Build history of the part. All positions in model axes, mm. Face numbers are marked on the shaded views. A direction names the side the tool comes from. Round coordinates to 2 decimals unless told otherwise and drop trailing zeros. Loops run counter-clockwise (first coordinate to the right, second up) from the corner with the lowest first, then second, coordinate; pieces in that order, holes last. Notation, with made-up numbers: (-36, 75.25) - (18, 75.25) arc R36 ccw to (18, 110.25) - close; hole circle Ø8 at (80, -10). An arc over 180 degrees is marked (long way). Use a Markdown table: item, result.
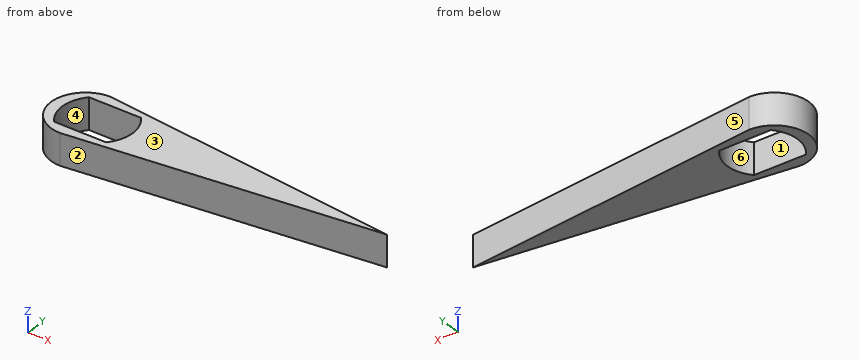
from build123d import *

# Parameters (mm, degrees)
PAD_DEPTH    = 2
POCKET_DEPTH = 2


with BuildPart() as part:
    # Sketch → Pad (new body)
    with BuildSketch(Plane(origin=(0, 0, 0), x_dir=(1, 0, 0), z_dir=(0, 0, -1))):
        with BuildLine():
            Line((0, 2.2), (19.5, 0))
            Line((19.5, 0), (0, -2.2))
            ThreePointArc((0, 2.2), (-2.2, 0), (0, -2.2))
        make_face()
    extrude(amount=PAD_DEPTH)

    # Sketch001 → Pocket (cut)
    with BuildSketch(Plane(origin=(0, 0, -2), x_dir=(1, 0, 0), z_dir=(0, 0, -1))):
        with BuildLine():
            Line((-0.899765, 1.5), (2.454335, 1.5))
            ThreePointArc((2.454335, -1.5), (3.027284, 0), (2.454335, 1.5))
            Line((-0.899765, -1.5), (2.454335, -1.5))
            ThreePointArc((-0.899765, 1.5), (-1.472714, 0), (-0.899765, -1.5))
        make_face()
    extrude(amount=-POCKET_DEPTH, mode=Mode.SUBTRACT)


solid = part.part
Q1. Pull direction Y, two halves, no side cores. Call the marked faces 3, 4, 5 and 6: pulls with the +Y half, pulls with the -Y half, needs draft (parallel to the pull), parting line crosses it, or undercut.
Results found:
| item | result |
|---|---|
| face 3 | needs draft |
| face 4 | undercut |
| face 5 | pulls with the +Y half |
| face 6 | undercut |
Q2. Cut at B-B, the plane y = 0.35. List the corners of the cut face in (x, z), plus the area to 3 significant figures.
Results found:
| item | result |
|---|---|
| outline | (-2.17, -2) - (-1.45, -2) - (-1.45, 0) - (-2.17, 0) - close; (3, -2) - (16.4, -2) - (16.4, 0) - (3, 0) - close |
| area | 28.2 mm2 |
Q3. Cut at D-D, the plane y = -0.6. List the corners of the cut face in (x, z), plus the area to 3 significant figures.
Results found:
| item | result |
|---|---|
| outline | (-2.12, -2) - (-1.39, -2) - (-1.39, 0) - (-2.12, 0) - close; (2.95, -2) - (14.18, -2) - (14.18, 0) - (2.95, 0) - close |
| area | 23.9 mm2 |
Q4. Probe line 1 (Y direction, x = 1, z = -1.3); line 2 (Y direction, x = 18.75, z = -1.75); line 3 (Y direction, x = 6.5, z = -0.05). List the from-to ranges inside material, lowest first.
Results found:
| item | result |
|---|---|
| line 1 | y = -2.09 to -1.5, 1.5 to 2.09 |
| line 2 | y = -0.08 to 0.08 |
| line 3 | y = -1.47 to 1.47 |
Q5. Cut at C-C, the plane y = 1.95. List the corners of the cut face in (x, z).
Results found:
| item | result |
|---|---|
| outline | (-1.02, -2) - (2.22, -2) - (2.22, 0) - (-1.02, 0) - close |
Q6. Cut at A-A, the plane z = -0.55. List the corners of the cut face in (x, y).
Results found:
| item | result |
|---|---|
| outline | (0, -2.2) - (19.5, 0) - (0, 2.2) arc R2.2 ccw to start; hole (-0.9, -1.5) - (2.45, -1.5) arc R2.25 ccw to (2.45, 1.5) - (-0.9, 1.5) arc R2.25 ccw to start |
Q7. Which spindle directions (+Z, -Z, +X, -X, +Y, -Y) get a long thin tool onto all of the face, cutting with end or side? Do the marked faces 1 and 2. Say none if no direction does.
Results found:
| item | result |
|---|---|
| face 1 | +Z, -Z |
| face 2 | +Z, -Z, +X, -Y |
